For this review, take the finished solid that the model builds, in its own axes (mm). A direction names the side the tool comes from. Round coordinates to 2 decimals unless told otherwise and drop trailing zeros. Order: outer loops, then holes, each group sorted by start corner. A loop starts at its lowest first (then second) coordinate and runs counter-clockwise, first axis right, second up. Notation, with made-up numbers: (-15, 57) -> (11, 57) arc R11 ccw to (11, 71) -> close; hole circle Ø8 at (-32, 78.25). An arc over 180 degrees is marked (long way). Use a Markdown table: item, result. Add a question column.
1) Consider section A-A (y = 50). State the section outline as (x, z) points.
2) Wall thickness on line 1 along Y through (x, z) = (-60, 1.5); line 2 along X through (y, z) = (47.5, 2.05); line 3 along Y through (x, z) = (-61.5, 2.1): over which ranges is each line inside the solid? List them lowest first. Write a range as [from, to].
3) Machinability: for faces 1 (the face through (-3.01, 22.85, 1.52)), 2 (the face through (-26, 17, 0)), which of the approach directions +Z, -Z, +X, -X, +Y, -Y give a long, thin tool a straight path to every point of the face, cutting with its end or side? Answer none if there is none.
4) Clearance check with a flat-ended pin moving along its axis: P1, Ø3.5, axis at x = -60, y = 30, coming from the +Z side. State where the tip first meets the part, or that it passes through.
5) Consider section D-D (y = 26.5). State the section outline as (x, z) points, plus the area to 3 significant figures.
6) Consider section C-C (x = -30). State the section outline as (y, z) points.
7) Draft analysis for pull direction X (two halves, no side actions). For faces 3 (the face through (-61.585, 31.453, 1.521)), 4 (the face through (10, 60, 1)), 5 (the face through (20, 34, 1)), 6 (the face through (10, 12, 2)), state which applies: pulls with the +X half, pulls with the -X half, needs draft (parallel to the pull), parting line crosses it, or undercut.
8) Consider section B-B (z = 1.55). Give the number of separate pieces and of enclosed holes in the cut face, plus the area to 3 significant figures.
```python
from build123d import *

# Parameters (mm, degrees)
SKETCH_1_W          = 20
SKETCH_1_H          = 60
EXTRUDE_1_DEPTH     = 3
SKETCH_2_W          = 60
SKETCH_2_H          = 20
EXTRUDE_2_DEPTH     = 3
SKETCH_3_R          = 2
CUT_EXTRUDE_1_DEPTH = 3
FILLET_1_R          = 10
SKETCH_4_W          = 20
SKETCH_4_H          = 60
SKETCH_4_W_2        = 10
SKETCH_4_H_2        = 20
EXTRUDE_3_DEPTH     = 3
SKETCH_5_R          = 2.15
CUT_EXTRUDE_2_DEPTH = 93.244241013
FILLET_3_R          = 10
FILLET_4_R          = 2


with BuildPart() as part:
    # 草图1 → 凸台-拉伸1 (new body)
    with BuildSketch(Plane.XY):
        with Locations((10, 30)):
            Rectangle(SKETCH_1_W, SKETCH_1_H)
    extrude(amount=EXTRUDE_1_DEPTH)

    # 草图2 → 凸台-拉伸2 (add)
    with BuildSketch(Plane.XY.offset(3)):
        with Locations((-10, 10)):
            Rectangle(SKETCH_2_W, SKETCH_2_H)
    extrude(amount=-EXTRUDE_2_DEPTH)

    # 草图3 → 切除-拉伸1 (cut)
    with BuildSketch(Plane.XY.offset(3)):
        with Locations((10, 10)):
            Circle(SKETCH_3_R)
        with Locations((10, 30)):
            Circle(SKETCH_3_R)
        with Locations((10, 50)):
            Circle(SKETCH_3_R)
        with Locations(Location((-10, 10, 0), (0, 0, 180))):
            Circle(SKETCH_3_R)
        with Locations(Location((-30, 10, 0), (0, 0, 180))):
            Circle(SKETCH_3_R)
    extrude(amount=-CUT_EXTRUDE_1_DEPTH, mode=Mode.SUBTRACT)

    # 圆角1
    fillet_1_edges = [part.edges().sort_by_distance(p)[0] for p in [
        (0, 20, 1.5),
        (20, 0, 1.5),
    ]]
    fillet(fillet_1_edges, radius=FILLET_1_R)

    # 草图4 → 凸台-拉伸3 (add, through all)
    with BuildSketch(Plane.XY.offset(3)):
        with Locations((-60, 30)):
            Rectangle(SKETCH_4_W, SKETCH_4_H)
        with Locations((-45, 10)):
            Rectangle(SKETCH_4_W_2, SKETCH_4_H_2)
    extrude(amount=-EXTRUDE_3_DEPTH)

    # 草图5 → 切除-拉伸2 (cut, through all)
    with BuildSketch(Plane.XY.offset(3)):
        with Locations((-60, 10)):
            Circle(SKETCH_5_R)
        with Locations((-60, 30)):
            Circle(SKETCH_5_R)
        with Locations((-60, 50)):
            Circle(SKETCH_5_R)
    extrude(amount=-CUT_EXTRUDE_2_DEPTH, mode=Mode.SUBTRACT)

    # 圆角3
    fillet_3_edges = [part.edges().sort_by_distance(p)[0] for p in [
        (-50, 20, 1.5),
        (-70, 0, 1.5),
    ]]
    fillet(fillet_3_edges, radius=FILLET_3_R)

    # 圆角4
    fillet_4_edges = [part.edges().sort_by_distance(p)[0] for p in [
        (-50, 60, 1.5),
        (-70, 60, 1.5),
        (0, 60, 1.5),
        (20, 60, 1.5),
    ]]
    fillet(fillet_4_edges, radius=FILLET_4_R)


solid = part.part
```
Results list:
| question | item | result |
|---|---|---|
| 1 | outline | (-70, 0) -> (-62.15, 0) -> (-62.15, 3) -> (-70, 3) -> close; (-57.85, 0) -> (-50, 0) -> (-50, 3) -> (-57.85, 3) -> close; (0, 0) -> (8, 0) -> (8, 3) -> (0, 3) -> close; (12, 0) -> (20, 0) -> (20, 3) -> (12, 3) -> close |
| 2 | line 1 | [0, 7.85], [12.15, 27.85], [32.15, 47.85], [52.15, 60] |
| 2 | line 2 | [-70, -50], [0, 20] |
| 2 | line 3 | [0.11, 8.46], [11.54, 28.46], [31.54, 48.46], [51.54, 60] |
| 3 | face 1 | +Z, -Z, +Y |
| 3 | face 2 | -Z, +X, -X, +Y, -Y |
| 4 | P1 | through |
| 5 | outline | (-70, 0) -> (-49.37, 0) -> (-49.37, 3) -> (-70, 3) -> close; (-0.63, 0) -> (20, 0) -> (20, 3) -> (-0.63, 3) -> close |
| 5 | area | 124 mm2 |
| 6 | outline | (0, 0) -> (8, 0) -> (8, 3) -> (0, 3) -> close; (12, 0) -> (20, 0) -> (20, 3) -> (12, 3) -> close |
| 7 | face 3 | undercut |
| 7 | face 4 | needs draft |
| 7 | face 5 | pulls with the +X half |
| 7 | face 6 | undercut |
| 8 | separate pieces | 1 |
| 8 | enclosed holes | 8 |
| 8 | area | 3,290 mm2 |
